from build123d import *

# Parameters (mm, degrees)
EXTRUDE_1_DEPTH      = 7.95
SKETCH_3_OUTSIDE_W   = 194.484
SKETCH_3_OUTSIDE_H   = 111.184
CUT_EXTRUDE_11_DEPTH = 0.001
SKETCH_5_R           = 1.056956527
CUT_EXTRUDE_12_DEPTH = 5
EXTRUDE_2_DEPTH      = 1
CUT_EXTRUDE_13_DEPTH = 5
SKETCH_8_R           = 0.78636109
CUT_EXTRUDE_14_DEPTH = 5
SKETCH_11_R          = 0.458710636
CUT_EXTRUDE_15_DEPTH = 5
EXTRUDE_3_DEPTH      = 3
SKETCH_14_R          = 8.784302199
SKETCH_14_R_2        = 5.477679508
EXTRUDE_4_DEPTH      = 2


with BuildPart() as part:
    # 草图1 → 凸台-拉伸1 (new body)
    with BuildSketch(Plane.XY):
        with BuildLine():
            Line((-68.8, 37.15), (68.8, 37.15))
            ThreePointArc((68.8, 37.15), (75.871067812, 34.221067812), (78.8, 27.15))
            Line((78.8, 27.15), (78.8, -27.15))
            ThreePointArc((78.8, -27.15), (75.871067812, -34.221067812), (68.8, -37.15))
            Line((68.8, -37.15), (-68.8, -37.15))
            ThreePointArc((-68.8, -37.15), (-75.871067812, -34.221067812), (-78.8, -27.15))
            Line((-78.8, -27.15), (-78.8, 27.15))
            ThreePointArc((-78.8, 27.15), (-75.871067812, 34.221067812), (-68.8, 37.15))
        make_face()
    extrude(amount=EXTRUDE_1_DEPTH)

    # 草图3 outside → 切除-拉伸11 (cut)
    with BuildSketch(Plane(origin=(0, 0, 0), x_dir=(-1, 0, 0), z_dir=(0, 0, -1))):
        Rectangle(SKETCH_3_OUTSIDE_W, SKETCH_3_OUTSIDE_H)
        with BuildLine():
            Line((-68.8, -36.1), (68.8, -36.1))
            ThreePointArc((68.8, -36.1), (75.128605692, -33.478605692), (77.75, -27.15))
            Line((77.75, -27.15), (77.75, 27.15))
            ThreePointArc((77.75, 27.15), (75.128605692, 33.478605692), (68.8, 36.1))
            Line((68.8, 36.1), (-68.8, 36.1))
            ThreePointArc((-68.8, 36.1), (-75.128605692, 33.478605692), (-77.75, 27.15))
            Line((-77.75, 27.15), (-77.75, -27.15))
            ThreePointArc((-77.75, -27.15), (-75.128605692, -33.478605692), (-68.8, -36.1))
        make_face(mode=Mode.SUBTRACT)
    extrude(amount=-CUT_EXTRUDE_11_DEPTH, mode=Mode.SUBTRACT)

    # 草图5 → 切除-拉伸12 (cut)
    with BuildSketch(Plane(origin=(78.8, 0, 0), x_dir=(0, 0, -1), z_dir=(1, 0, 0))):
        with Locations(Location((-3.9755, 24.926367293, 0), (0, 0, 90))):
            Circle(SKETCH_5_R)
    extrude(amount=-CUT_EXTRUDE_12_DEPTH, mode=Mode.SUBTRACT)

    # 草图6 → 凸台-拉伸2 (add)
    with BuildSketch(Plane(origin=(0, 37.15, 0), x_dir=(1, 0, 0), z_dir=(0, 1, 0))):
        with BuildLine():
            Line((36.881407925, -2.384573788), (57.653695148, -2.384573788))
            ThreePointArc((57.653695148, -2.384573788), (59.24462136, -3.9755), (57.653695148, -5.566426212))
            Line((57.653695148, -5.566426212), (36.881407925, -5.566426212))
            ThreePointArc((36.881407925, -5.566426212), (35.290481714, -3.9755), (36.881407925, -2.384573788))
        make_face()
        with BuildLine():
            Line((30.204601318, -5.24848304), (18.54668502, -5.24848304))
            ThreePointArc((18.54668502, -5.24848304), (17.27370198, -3.9755), (18.54668502, -2.70251696))
            Line((18.54668502, -2.70251696), (30.204601318, -2.70251696))
            ThreePointArc((30.204601318, -2.70251696), (31.477584358, -3.9755), (30.204601318, -5.24848304))
        make_face()
    extrude(amount=EXTRUDE_2_DEPTH)

    # 草图7 → 切除-拉伸13 (cut)
    with BuildSketch(Plane.ZY.offset(78.8)):
        with BuildLine():
            Line((3.210974453, -3.219498771), (3.210974453, 3.219498771))
            ThreePointArc((3.210974453, 3.219498771), (3.9755, 3.984024318), (4.740025547, 3.219498771))
            Line((4.740025547, 3.219498771), (4.740025547, -3.219498771))
            ThreePointArc((4.740025547, -3.219498771), (3.9755, -3.984024318), (3.210974453, -3.219498771))
        make_face()
    extrude(amount=-CUT_EXTRUDE_13_DEPTH, mode=Mode.SUBTRACT)

    # 草图8 → 切除-拉伸14 (cut)
    with BuildSketch(Plane.ZY.offset(78.8)):
        with Locations(Location((3.9755, 25.237609302, 0), (0, 0, 270))):
            Circle(SKETCH_8_R)
        with Locations(Location((3.9755, 22.616405668, 0), (0, 0, 270))):
            Circle(SKETCH_8_R)
        with Locations(Location((3.9755, 19.995202033, 0), (0, 0, 270))):
            Circle(SKETCH_8_R)
        with Locations(Location((3.9755, 17.570588671, 0), (0, 0, 270))):
            Circle(SKETCH_8_R)
        with Locations(Location((3.9755, 15.145975309, 0), (0, 0, 270))):
            Circle(SKETCH_8_R)
        with Locations(Location((3.9755, 12.590301765, 0), (0, 0, 270))):
            Circle(SKETCH_8_R)
    extrude(amount=-CUT_EXTRUDE_14_DEPTH, mode=Mode.SUBTRACT)

    # 草图11 → 切除-拉伸15 (cut)
    with BuildSketch(Plane.ZY.offset(78.8)):
        with Locations(Location((3.9755, -25.155030575, 0), (0, 0, 270))):
            Circle(SKETCH_11_R)
    extrude(amount=-CUT_EXTRUDE_15_DEPTH, mode=Mode.SUBTRACT)

    # 草图13 → 凸台-拉伸3 (add)
    with BuildSketch(Plane.XY.offset(7.95)):
        with BuildLine():
            Line((35.665823079, 33.513099336), (60.458995853, 33.513099336))
            ThreePointArc((60.458995853, 33.513099336), (69.352474106, 28.08541216), (68.591748787, 17.694308248))
            Line((68.591748787, 17.694308248), (56.1951624, 0.367964546))
            ThreePointArc((56.1951624, 0.367964546), (48.062409466, -3.813244367), (39.929656532, 0.367964546))
            Line((39.929656532, 0.367964546), (27.533070145, 17.694308248))
            ThreePointArc((27.533070145, 17.694308248), (26.772344826, 28.08541216), (35.665823079, 33.513099336))
        make_face()
    extrude(amount=EXTRUDE_3_DEPTH)

    # 草图14 → 凸台-拉伸4 (add)
    with BuildSketch(Plane.XY.offset(10.95)):
        with Locations(Location((48.062409466, 8.713531937, 0), (0, 0, 180))):
            Circle(SKETCH_14_R)
        with Locations(Location((35.665823079, 23.513099336, 0), (0, 0, 180))):
            Circle(SKETCH_14_R_2)
        with Locations(Location((60.458995853, 23.513099336, 0), (0, 0, 180))):
            Circle(SKETCH_14_R_2)
    extrude(amount=EXTRUDE_4_DEPTH)


solid = part.part
Work out the finished part from the listing and answer in its coordinate system (mm). A direction names the side the tool comes from. Round coordinates to 2 decimals unless told otherwise and drop trailing zeros.
1) A tool of negligible diameter and unlimited length cuts with its end or side. For faces 5 (the cylindrical face through (48.195, -3.812, 9.429)), 6 (the flat face through (33.82, 8.91, 9.43)), 7 (the cylindrical face through (26.703, 27.948, 9.429)), 8 (the cylindrical face through (39.95, 12.08, 11.94)), from which of +Z, -Z, +X, -X, +Y, -Y can it reach the whole face along a straight path? Write none if from no direction.
2) Given pin 1 Ø0.6 at (y, z) = (25, 3.5) entering from +X; pin 2 Ø6.5 at (x, z) = (3.5, 4) entering from +Y; pin 3 Ø0.9 at (x, z) = (46, 8.5) entering from +Y, each flat-ended and moving along its own axis, determine where each tip first touches the part or whether it passes through.
3) Straight lines are drawn through the part: line 1 (Z direction, x = 69, y = 30.5); line 2 (Y direction, x = -62, z = 3); line 3 (Y direction, x = 48.5, z = 12.75). For each, find the intervals that lie inside material, in ascending order.
4) The mould has two halves that part along Y. Classify faces 1 (the cylindrical face through (-75.79, -34.3, 3.92)), 2 (the cylindrical face through (75.79, 34.3, 3.92)), 3 (the flat face through (78.8, 0, 4)), 4 (the flat face through (-76, 0, 4.74)): pulls with the +Y half, pulls with the -Y half, needs draft (parallel to the pull), parting line crosses it, or undercut.
Completed:
1. face 5: +Z, -Y
1. face 6: +Z, -X, -Y
1. face 7: +Z, -X
1. face 8: +Z
2. pin 1: stops at x = 73.8
2. pin 2: stops at y = 37.15
2. pin 3: stops at y = 33.51
3. line 1: z = 0 to 7.95
3. line 2: y = -37.15 to 37.15
3. line 3: y = -0.06 to 17.49
4. face 1: pulls with the -Y half
4. face 2: pulls with the +Y half
4. face 3: needs draft
4. face 4: undercut
